Autodesk Inventor part; units mm, degrees
ref_plane "YZ Plane" through (0, 0, 0) normal (1, 0, 0) x (0, 1, 0)
ref_plane "XZ Plane" through (0, 0, 0) normal (0, 1, 0) x (-1, 0, 0)
ref_plane "XY Plane" through (0, 0, 0) normal (0, 0, 1) x (1, 0, 0)
ref_plane "Arbeitsebene1" through (0, 0, 0) normal (0, 0, 1) x (1, 0, 0)
sketch "Skizze1" plane through (0, 0, 0) normal (0, 0, 1) x (1, 0, 0)
  circle A0 centre (0, -25) radius 2.5
  circle A1 centre (0, 25) radius 2.5
  line L0 (12.5, -37) -> (12.5, 37)
  line L1 (12.5, 37) -> (-12.5, 37)
  line L2 (-12.5, 37) -> (-12.5, -37)
  line L3 (-12.5, -37) -> (12.5, -37)
  circle A2 centre (8.5, -30) radius 1.4
  circle A3 centre (-8.5, -30) radius 1.4
  circle A4 centre (-8.5, 30) radius 1.4
  circle A5 centre (8.5, 30) radius 1.4
  circle A6 centre (0, 0) radius 6
  circle A7 centre (0, 25) radius 2.7
  circle A8 centre (0, -25) radius 2.7
  line L4 (-9.25, 9.25) -> (9.25, 9.25)
  line L5 (9.25, 9.25) -> (9.25, -9.25)
  line L6 (9.25, -9.25) -> (-9.25, -9.25)
  line L7 (-9.25, -9.25) -> (-9.25, 9.25)
  point P0 (0.75, -9.25)
  point P1 (-0.75, -9.25)
  point P2 (-0.75, 9.25)
  point P3 (0.75, 9.25)
  point P4 (0.75, 5.9529)
  point P5 (-0.75, 5.9529)
  point P6 (0.75, -5.9529)
  point P7 (-0.75, -5.9529)
  dimension "d0" = 12
  dimension "d4" = 0.2
  dimension "d5" = 0.2
extrude "Extrusion1" add sketch "Skizze1" along normal blind 2 contours L3 L2 L1 L0 | L4 L5 L6 L7
sketch "Skizze2" plane through (0, 0, 0) normal (0, 0, -1) x (-1, 0, 0)
  line L0 (-9, -9) -> (-9, 9)
  line L1 (9, -9) -> (-9, -9)
  line L2 (9, 9) -> (9, -9)
  line L3 (-9, 9) -> (9, 9)
  line L4 (9.5, -9.5) -> (-9.5, -9.5)
  line L5 (-9.5, -9.5) -> (-9.5, 9.5)
  line L6 (-9.5, 9.5) -> (9.5, 9.5)
  line L7 (9.5, 9.5) -> (9.5, -9.5)
  point P0 (0, 0)
  dimension "d6" = 0.5
properties part number "40_microfluidic_chip_lightsheet_layer2_v0"
Check sheet for the modelled part. Datum: model origin and axes. Units: mm. Round coordinates to 2 decimals unless told otherwise and drop trailing zeros. Order: outer loops, then holes, each group sorted by start corner. A loop starts at its lowest first (then second) coordinate and runs counter-clockwise, first axis right, second up. Notation, with made-up numbers: M 84,-24.75 L 132,-24.75 A32 cw 132,1.25 Z; hole C 51.5,31 d5. An arc over 180 degrees is marked long. One line per item, written item: value. Start each with the question number.
1. Gauge pin test, flat end, axial feed: P1, Ø6, axis at x = 0, y = 12.5, coming from the -Z side. Record the tip position at first contact, or that the pin passes through.
2. Section check D-D on z = 0.55. Enter the section's corners in (x, y), and give its area (3 significant figures).
3. Section check B-B on x = 0. Enter the section's corners in (y, z).
4. Section check C-C on x = 8.5. Enter the section's corners in (y, z).
5. Release check for a two-part mould opening along Y. For faces 1 (the flat face through (0, -37, 1)), 2 (the flat face through (12.5, -1, 1)), 3 (the cylindrical face through (8.32, 28.61, 0.99)) record: released by +Y, released by -Y, zero draft, split by the parting line, or undercut.
6. Section check A-A on y = 0. Enter the section's corners in (x, z), and give its area (3 significant figures).
7. Scan lines: line 1 along Y through (x, z) = (0, 0.65); line 2 along Y through (x, z) = (8.5, 1.55); line 3 along Y through (x, z) = (8, 0.55). Record each from-to range of solid material in increasing order.
Results found:
1. P1: z = 0
2. outline: M -12.5,-37 L 12.5,-37 L 12.5,37 L -12.5,37 Z; hole C -8.5,-30 d2.8; hole C -8.5,30 d2.8; hole C 0,0 d12; hole C 0,-25 d5.4; hole C 0,25 d5.4; hole C 8.5,-30 d2.8; hole C 8.5,30 d2.8
2. area: 1,670 mm^2
3. outline: M -37,0 L -27.7,0 L -27.7,2 L -37,2 Z; M -22.3,0 L -6,0 L -6,2 L -22.3,2 Z; M 6,0 L 22.3,0 L 22.3,2 L 6,2 Z; M 27.7,0 L 37,0 L 37,2 L 27.7,2 Z
4. outline: M -37,0 L -31.4,0 L -31.4,2 L -37,2 Z; M -28.6,0 L 28.6,0 L 28.6,2 L -28.6,2 Z; M 31.4,0 L 37,0 L 37,2 L 31.4,2 Z
5. face 1: released by -Y
5. face 2: zero draft
5. face 3: undercut
6. outline: M -12.5,0 L -6,0 L -6,2 L -12.5,2 Z; M 6,0 L 12.5,0 L 12.5,2 L 6,2 Z
6. area: 26.0 mm^2
7. line 1: -37 to -27.7, -22.3 to -6, 6 to 22.3, 27.7 to 37
7. line 2: -37 to -31.4, -28.6 to 28.6, 31.4 to 37
7. line 3: -37 to -31.31, -28.69 to 28.69, 31.31 to 37
